```python
from build123d import *

# Parameters (mm, degrees)
SKETCH_R     = 1.6
PAD_DEPTH    = 2.8
PAD001_DEPTH = 13
FILLET_R     = 2
SKETCH002_R  = 1.6
HOLE_DEPTH   = 68.401
FILLET001_R  = 3
POCKET_DEPTH = 2.8


with BuildPart() as part:
    # Sketch → Pad (new body)
    with BuildSketch(Plane.XY):
        with BuildLine():
            Line((26.35, 26.7), (26.35, -26.7))
            ThreePointArc((24.35, -28.7), (25.764214, -28.114214), (26.35, -26.7))
            Line((24.35, -28.7), (-24.35, -28.7))
            ThreePointArc((-26.35, -26.7), (-25.764214, -28.114214), (-24.35, -28.7))
            Line((-26.35, -26.7), (-26.35, 26.7))
            ThreePointArc((-26.072403, 27.716527), (-26.279353, 27.226875), (-26.35, 26.7))
            Line((-26.072403, 27.716527), (-19, 39.7))
            Line((-19, 39.7), (19, 39.7))
            Line((26.072403, 27.716527), (19, 39.7))
            ThreePointArc((26.35, 26.7), (26.279353, 27.226875), (26.072403, 27.716527))
        make_face()
        with Locations((-18.75, -22.2)):
            Circle(SKETCH_R, mode=Mode.SUBTRACT)
        with Locations((18.75, -22.2)):
            Circle(SKETCH_R, mode=Mode.SUBTRACT)
        with Locations((18.75, 22.2)):
            Circle(SKETCH_R, mode=Mode.SUBTRACT)
        with Locations((-18.75, 22.2)):
            Circle(SKETCH_R, mode=Mode.SUBTRACT)
        with BuildLine():
            Line((-15.75, 36.9), (15.75, 36.9))
            Line((15.75, 22.2), (15.75, 36.9))
            ThreePointArc((15.75, 22.2), (16.62868, 20.07868), (18.75, 19.2))
            Line((22.35, 19.2), (18.75, 19.2))
            ThreePointArc((23.35, 18.2), (23.057107, 18.907107), (22.35, 19.2))
            Line((23.35, 18.2), (23.35, -18.2))
            ThreePointArc((22.35, -19.2), (23.057107, -18.907107), (23.35, -18.2))
            Line((22.35, -19.2), (18.75, -19.2))
            ThreePointArc((18.75, -19.2), (16.62868, -20.07868), (15.75, -22.2))
            Line((15.75, -22.2), (15.75, -24.7))
            ThreePointArc((14.75, -25.7), (15.457107, -25.407107), (15.75, -24.7))
            Line((14.75, -25.7), (-14.75, -25.7))
            ThreePointArc((-15.75, -24.7), (-15.457107, -25.407107), (-14.75, -25.7))
            Line((-15.75, -22.2), (-15.75, -24.7))
            ThreePointArc((-15.75, -22.2), (-16.62868, -20.07868), (-18.75, -19.2))
            Line((-22.35, -19.2), (-18.75, -19.2))
            ThreePointArc((-23.35, -18.2), (-23.057107, -18.907107), (-22.35, -19.2))
            Line((-23.35, -18.2), (-23.35, 18.2))
            ThreePointArc((-22.35, 19.2), (-23.057107, 18.907107), (-23.35, 18.2))
            Line((-22.35, 19.2), (-18.75, 19.2))
            ThreePointArc((-18.75, 19.2), (-16.62868, 20.07868), (-15.75, 22.2))
            Line((-15.75, 22.2), (-15.75, 36.9))
        make_face(mode=Mode.SUBTRACT)
    extrude(amount=PAD_DEPTH)

    # Sketch001 (on Face37 of Pad) → Pad001 (join)
    with BuildSketch(Plane(origin=(0, 0, 0), x_dir=(1, 0, 0), z_dir=(0, 0, -1))):
        Polygon((-20.652503, -36.9), (20.652503, -36.9), (19, -39.7), (-19, -39.7), align=None)
    extrude(amount=PAD001_DEPTH)

    # Fillet
    fillet_edges = [part.edges().sort_by_distance(p)[0] for p in [
        (-18.201252, 36.9, 0),
        (18.201252, 36.9, 0),
    ]]
    fillet(fillet_edges, radius=FILLET_R)

    # Sketch002 (on Face45 of Fillet) → Hole (cut, through all)
    with BuildSketch(Plane(origin=(0, 39.7, 0), x_dir=(-1, 0, 0), z_dir=(0, 1, 0))):
        with Locations((-10.75, -9)):
            Circle(SKETCH002_R)
        with Locations((10.75, -9)):
            Circle(SKETCH002_R)
    extrude(amount=-HOLE_DEPTH, mode=Mode.SUBTRACT)

    # Fillet001
    fillet001_edges = [part.edges().sort_by_distance(p)[0] for p in [
        (-19.826252, 38.3, -13),
        (19.826252, 38.3, -13),
    ]]
    fillet(fillet001_edges, radius=FILLET001_R)

    # Sketch003 (on Face5 of Fillet001) → Pocket (cut)
    with BuildSketch(Plane(origin=(0, 39.7, 0), x_dir=(-1, 0, 0), z_dir=(0, 1, 0))):
        with BuildLine():
            Line((-15.75, 2.8), (15.75, 2.8))
            Line((15.75, 2.8), (15.75, -4))
            ThreePointArc((14.75, -5), (15.457107, -4.707107), (15.75, -4))
            Line((14.75, -5), (-14.75, -5))
            ThreePointArc((-15.75, -4), (-15.457107, -4.707107), (-14.75, -5))
            Line((-15.75, -4), (-15.75, 2.8))
        make_face()
    extrude(amount=-POCKET_DEPTH, mode=Mode.SUBTRACT)


solid = part.part
```
Can you work these out from the model? Positions are in its coordinate system, mm. A direction names the side the tool comes from. Coordinates: 2 decimals unless noted, no trailing zeros. Order: outer loops, then holes, each group sorted by start corner. A loop starts at its lowest first (then second) coordinate and runs counter-clockwise, first axis right, second up. Notation, with made-up numbers: (26.25, 22.25) - (32.25, 22.25) arc R30 cw to (32.25, 57.25) - close; hole circle Ø2 at (28, -3). An arc over 180 degrees is marked (long way). Answer in a Markdown table with one row per item.
1. Suppose I cut it at B-B (z = -9). Please give me the cut outline in (x, y), and give its area (3 significant figures).
Reply:
| item | result |
|---|---|
| outline | (-20.65, 36.9) - (-12.35, 36.9) - (-12.35, 39.7) - (-19, 39.7) - close; (-9.15, 36.9) - (9.15, 36.9) - (9.15, 39.7) - (-9.15, 39.7) - close; (12.35, 36.9) - (20.65, 36.9) - (19, 39.7) - (12.35, 39.7) - close |
| area | 93.1 mm^2 |
2. Suppose I cut it at D-D (x = 10.75). Please give me the cut outline in (y, z), and give its area (3 significant figures).
Reply:
| item | result |
|---|---|
| outline | (-28.7, 0) - (-25.7, 0) - (-25.7, 2.8) - (-28.7, 2.8) - close; (36.9, -13) - (39.7, -13) - (39.7, -10.6) - (36.9, -10.6) - close; (36.9, -7.4) - (39.7, -7.4) - (39.7, -5) - (36.9, -5) - close |
| area | 21.8 mm^2 |
3. If we mould it in two halves opening along X, with no side actions, what happens to faces 5 (the cylindrical face through (-9.5, 38.3, -10)), 6 (the flat face through (21, -19.2, 1)), 7 (the flat face through (0, -28.7, 1)), 8 (the flat face through (26.35, 0, 1))? For each: pulls with the +X half, pulls with the -X half, needs draft (parallel to the pull), parting line crosses it, or undercut.
Reply:
| item | result |
|---|---|
| face 5 | undercut |
| face 6 | undercut |
| face 7 | needs draft |
| face 8 | pulls with the +X half |
4. If I drill on line 1 along Y through (x, z) = (-18.75, 1.2); line 2 along Y through (x, z) = (-17.5, 0.5); line 3 along X through (y, z) = (-3, 0.5), over which ranges is the centre line in solid material (lowest first)?
Reply:
| item | result |
|---|---|
| line 1 | y = -28.7 to -23.8, -20.6 to -19.2, 19.2 to 20.6, 23.8 to 39.7 |
| line 2 | y = -28.7 to -23.2, -21.2 to -19.47, 19.47 to 21.2, 23.2 to 39.7 |
| line 3 | x = -26.35 to -23.35, 23.35 to 26.35 |
5. For faces 1 (the flat face through (-15.75, 33, 1)), 2 (the flat face through (0, 38, -5)), 3 (the cylindrical face through (-16.61, -20.1, 1.38)), 4 (the flat face through (0, -25.7, 1)), which set-ups out of +Z, -Z, +X, -X, +Y, -Y let a thin tool reach every point of the face, with its end or its side?
Reply:
| item | result |
|---|---|
| face 1 | +Z, +Y |
| face 2 | +Z, +Y, -Y |
| face 3 | +Z, -Z |
| face 4 | +Z, -Z, +Y |
6. Suppose I cut it at C-C (y = -4). Please give me the cut outline in (x, z), and give its area (3 significant figures).
Reply:
| item | result |
|---|---|
| outline | (-26.35, 0) - (-23.35, 0) - (-23.35, 2.8) - (-26.35, 2.8) - close; (23.35, 0) - (26.35, 0) - (26.35, 2.8) - (23.35, 2.8) - close |
| area | 16.8 mm^2 |
7. For pin 1 (1.4 mm diameter, centred on x = 20.5, z = 2, fed in from +Y); pin 2 (3.5 mm diameter, centred on x = -18.75, y = 22.2, fed in from -Z); pin 3 (5 mm diameter, centred on x = -10.75, z = -9, fed in from +Y); pin 4 (7.5 mm diameter, centred on y = 35, z = 0, fed in from +X), each with a flat end and sliding along its axis, tell me the tip position at first contact or that it passes through.
Reply:
| item | result |
|---|---|
| pin 1 | stops at y = 38.34 |
| pin 2 | stops at z = 0 |
| pin 3 | stops at y = 39.7 |
| pin 4 | stops at x = 23.99 |
8. Suppose I cut it at A-A (x = 4.5). Please give me the cut outline in (y, z), and give its area (3 significant figures).
Reply:
| item | result |
|---|---|
| outline | (-28.7, 0) - (-25.7, 0) - (-25.7, 2.8) - (-28.7, 2.8) - close; (36.9, -13) - (39.7, -13) - (39.7, -5) - (36.9, -5) - close |
| area | 30.8 mm^2 |
